Part model, mm, in its own coordinate system. A direction names the side the tool comes from. Give positions to 0.01 mm unless a question says otherwise; leave off trailing zeros. Order: outer loops, then holes, each group sorted by start corner. A loop starts at its lowest first (then second) coordinate and runs counter-clockwise, first axis right, second up. Notation, with made-up numbers: M 52.5,36.5 L 97.5,36.5 A4 cw 97.5,41.5 Z; hole C -38,59 d7. An arc over 180 degrees is marked long. Return JSON: item names as keys, results as strings.
from build123d import *

# Parameters (mm, degrees)
ESQUISSE1_R              = 5
BOSS_EXTRU_1_DEPTH       = 8
ESQUISSE2_R              = 7.5
BOSS_EXTRU_3_DEPTH       = 2
ESQUISSE5_R              = 7.25
BOSS_EXTRU_6_DEPTH       = 1
ESQUISSE8_R              = 7.5
BOSS_EXTRU_8_DEPTH       = 9
ESQUISSE9_R              = 7.25
BOSS_EXTRU_9_DEPTH       = 1
ESQUISSE10_R             = 7.5
BOSS_EXTRU_10_DEPTH      = 11
ESQUISSE11_R             = 6
BOSS_EXTRU_11_DEPTH      = 23
ESQUISSE12_R             = 4.5
BOSS_EXTRU_12_DEPTH      = 11
ENL_V_START              = 6
ENL_V_MAT_EXTRU_7_DEPTH  = 5
ENL_V_START_2            = 4
ENL_V_MAT_EXTRU_9_DEPTH  = 5
ESQUISSE17_R             = 2.25
ENL_V_MAT_EXTRU_10_DEPTH = 5


with BuildPart() as part:
    # Esquisse1 → Boss.-Extru.1 (new body)
    with BuildSketch(Plane.XY):
        Circle(ESQUISSE1_R)
    extrude(amount=BOSS_EXTRU_1_DEPTH)

    # Esquisse2 → Boss.-Extru.3 (add)
    with BuildSketch(Plane.XY):
        Circle(ESQUISSE2_R)
    extrude(amount=-BOSS_EXTRU_3_DEPTH)

    # Esquisse5 → Boss.-Extru.6 (add)
    with BuildSketch(Plane(origin=(0, 0, -2), x_dir=(-1, 0, 0), z_dir=(0, 0, -1))):
        with Locations(Location((0, 0, 0), (0, 0, 180))):  # turned: the seam where the file's is
            Circle(ESQUISSE5_R)
    extrude(amount=BOSS_EXTRU_6_DEPTH)

    # Esquisse8 → Boss.-Extru.8 (add)
    with BuildSketch(Plane(origin=(0, 0, -3), x_dir=(-1, 0, 0), z_dir=(0, 0, -1))):
        with Locations(Location((0, 0, 0), (0, 0, 180))):  # turned: the seam where the file's is
            Circle(ESQUISSE8_R)
    extrude(amount=BOSS_EXTRU_8_DEPTH)

    # Esquisse9 → Boss.-Extru.9 (add)
    with BuildSketch(Plane(origin=(0, 0, -12), x_dir=(-1, 0, 0), z_dir=(0, 0, -1))):
        with Locations(Location((0, 0, 0), (0, 0, 180))):  # turned: the seam where the file's is
            Circle(ESQUISSE9_R)
    extrude(amount=BOSS_EXTRU_9_DEPTH)

    # Esquisse10 → Boss.-Extru.10 (add)
    with BuildSketch(Plane(origin=(0, 0, -13), x_dir=(-1, 0, 0), z_dir=(0, 0, -1))):
        with Locations(Location((0, 0, 0), (0, 0, 180))):  # turned: the seam where the file's is
            Circle(ESQUISSE10_R)
    extrude(amount=BOSS_EXTRU_10_DEPTH)

    # Esquisse11 → Boss.-Extru.11 (add)
    with BuildSketch(Plane(origin=(0, 0, -24), x_dir=(-1, 0, 0), z_dir=(0, 0, -1))):
        Circle(ESQUISSE11_R)
    extrude(amount=BOSS_EXTRU_11_DEPTH)

    # Esquisse12 → Boss.-Extru.12 (add)
    with BuildSketch(Plane(origin=(0, 0, -47), x_dir=(-1, 0, 0), z_dir=(0, 0, -1))):
        Circle(ESQUISSE12_R)
    extrude(amount=BOSS_EXTRU_12_DEPTH)

    # Esquisse14 → Enlèv. mat.-Extru.7 (cut)
    with BuildSketch(Plane(origin=(0, 0, 0), x_dir=(1, 0, 0), z_dir=(0, 1, 0)).offset(ENL_V_START)):
        with BuildLine():
            Line((-1.5, 4.65), (-1.5, 10.3))
            ThreePointArc((-1.5, 10.3), (0, 11.8), (1.5, 10.3))
            Line((1.5, 10.3), (1.5, 4.65))
            ThreePointArc((1.5, 4.65), (0, 3.15), (-1.5, 4.65))
        make_face()
    extrude(amount=ENL_V_MAT_EXTRU_7_DEPTH, mode=Mode.SUBTRACT)

    # Esquisse15 → Enlèv. mat.-Extru.9 (cut)
    with BuildSketch(Plane(origin=(0, 0, 0), x_dir=(1, 0, 0), z_dir=(0, 1, 0)).offset(ENL_V_START_2)):
        with BuildLine():
            Line((-1, 48.15), (-1, 56.65))
            ThreePointArc((-1, 56.65), (0, 57.65), (1, 56.65))
            Line((1, 56.65), (1, 48.15))
            ThreePointArc((1, 48.15), (0, 47.15), (-1, 48.15))
        make_face()
    extrude(amount=ENL_V_MAT_EXTRU_9_DEPTH, mode=Mode.SUBTRACT)

    # Esquisse17 → Enlèv. mat.-Extru.10 (cut)
    with BuildSketch(Plane(origin=(0, 0, -58), x_dir=(-1, 0, 0), z_dir=(0, 0, -1))):
        Circle(ESQUISSE17_R)
    extrude(amount=-ENL_V_MAT_EXTRU_10_DEPTH, mode=Mode.SUBTRACT)


solid = part.part
Q1. Probe line 1 along Y through (x, z) = (0, -54.6); line 2 along Z through (x, y) = (-2.25, -5.25); line 3 along X through (y, z) = (-0.25, -15). List the from-to ranges inside material, lowest first.
Established:
{"line 1": "y = -4.5 to -2.25, 2.25 to 4", "line 2": "z = -47 to 0", "line 3": "x = -7.5 to 7.5"}
Q2. Band-saw the part on B-B (z = -32.5). Give the cut face in (x, y).
Established:
{"outline": "C 0,0 d12"}
Q3. Pin check, flat tips, straight feed: pin 1 (1.5 mm diameter, centred on y = 7, z = -8.5, fed in from -X); pin 2 (6 mm diameter, centred on y = 2.5, z = -26.5, fed in from +X); pin 3 (3 mm diameter, centred on y = 2.5, z = -44, fed in from +X). Stop position of each tip, or through.
Established:
{"pin 1": "stops at x = -4.15", "pin 2": "stops at x = 7.45", "pin 3": "stops at x = 5.92"}
Q4. Band-saw the part on A-A (z = 2). Give the cut face in (x, y).
Established:
{"outline": "C 0,0 d10"}
Q5. Band-saw the part on C-C (z = -6). Give the cut face in (x, y), then the cut area to 3 significant figures.
Established:
{"outline": "M -1.5,6 L -1.5,7.35 A7.5 ccw long 1.5,7.35 L 1.5,6 Z", "area": "172 mm²"}
Q6. Two-plate mould, pull along Z, no slides. Class faces 5 (the flat face through (2, -6, -24)), 6 (the cylindrical face through (0.03, 6.74, -3.15)), 7 (the cylindrical face through (3.35, 6.43, -2.49)), 8 (the cylindrical face through (-7.493, 0.33, -0.986)): +Z half, -Z half, draft (parallel to the pull), parting line (faces both ways), or undercut.
Established:
{"face 5": "-Z half", "face 6": "undercut", "face 7": "undercut", "face 8": "draft"}
Q7. 3-axis set-ups, long thin cutter, end or side, ignore diameter. For faces 1 (the cylindrical face through (3.35, 6.43, -12.49)), 2 (the flat face through (0, 4, -52)), 3 (the cylindrical face through (0.29, 2.23, -55.54)), 4 (the cylindrical face through (-1.08, -4.88, 3.94)): which of +Z, -Z, +X, -X, +Y, -Y reach the whole face in a straight line?
Established:
{"face 1": "none", "face 2": "+Y", "face 3": "-Z", "face 4": "+Z"}
